Source: CAD feature listing. Evaluate the final solid. Frame: model axes, mm. A direction names the side the tool comes from. Coordinates: 2 decimals unless noted, no trailing zeros. Order: outer loops, then holes, each group sorted by start corner. A loop starts at its lowest first (then second) coordinate and runs counter-clockwise, first axis right, second up. Notation, with made-up numbers: (-30.75, 74) -> (-19.75, 74) arc R31 cw to (-19.75, 112) -> close; hole circle Ø4 at (43, 71.25). An arc over 180 degrees is marked (long way). Write item = value, one per line. Start each with the question number.
Item 1: Section query B-B (x = -25). Output: boundary loops of the cut face in (y, z), then the cut area to 3 significant figures.
Item 2: Contact query for flat-ended pins moving along their axis: pin 1 (6 mm diameter, centred on x = -17, y = 3, fed in from +Z); pin 2 (10 mm diameter, centred on x = -20, z = 10, fed in from +Y); pin 3 (2 mm diameter, centred on x = -26.5, y = 14, fed in from -Z); pin 4 (12 mm diameter, centred on x = -16.5, y = -53.5, fed in from -Z). Output: stop coordinate, or through.
Item 3: Section query C-C (y = -35). Output: boundary loops of the cut face in (x, z).
Item 4: Ray query, line 1 along Y through (x, z) = (-16.75, 6.75); line 2 along X through (y, z) = (-69.3, 10.05); line 3 along Z through (x, y) = (-19.25, 26.5). Return the intervals inside material, ascending. Write a range as [from, to].
Item 5: Section query A-A (z = 6). Output: boundary loops of the cut face in (x, y).
Item 6: Set-up query: faces 1 (the flat face through (-12.21, -34, 10)), 2 (the cylindrical face through (-19.95, -39.68, 1.97)), 3 (the flat face through (-17, -55, 20.1)). Return all of +Z, -Z, +X, -X, +Y, -Y with unobstructed straight access to the full face (end or side cutting, diameter ignored); none if empty.
Item 7: Mould query, pull axis X, two halves, no side actions, for faces 4 (the cylindrical face through (-21.61, -58.31, 22.07)), 5 (the flat face through (-19, -69, 0)), 6 (the flat face through (-29.21, -27, 3)), 7 (the cylindrical face through (-20.41, -45.29, 12.4)). Classes: released by +X, released by -X, zero draft, split by the parting line, or undercut.
Item 8: Section query D-D (y = 0). Output: boundary loops of the cut face in (x, z).
```python
from build123d import *

# Parameters (mm, degrees)
SKETCH_1_W          = 20
SKETCH_1_H          = 90
EXTRUDE_1_DEPTH     = 4
SKETCH_2_W          = 20
SKETCH_2_H          = 4
EXTRUDE_2_DEPTH     = 20.1
SKETCH_3_W          = 20
SKETCH_3_H          = 4
EXTRUDE_3_DEPTH     = 24.1
SKETCH_4_W          = 20
SKETCH_4_H          = 4
EXTRUDE_4_DEPTH     = 20.1
SKETCH_5_R          = 2.6
CUT_EXTRUDE_1_DEPTH = 20
SKETCH_6_R          = 2.6
CUT_EXTRUDE_2_DEPTH = 20
SKETCH_7_R          = 2.6
CUT_EXTRUDE_3_DEPTH = 20
SKETCH_9_R          = 1.6
CUT_EXTRUDE_4_DEPTH = 20
EXTRUDE_5_DEPTH     = 3


with BuildPart() as part:
    # 草图1 → 凸台-拉伸1 (new body)
    with BuildSketch(Plane.XY):
        with Locations((-19.209677061, -2.260885663)):
            Rectangle(SKETCH_1_W, SKETCH_1_H)
    extrude(amount=EXTRUDE_1_DEPTH)

    # 草图2 → 凸台-拉伸2 (add)
    with BuildSketch(Plane.XY.offset(4)):
        with Locations((-19.209677061, -45.260885663)):
            Rectangle(SKETCH_2_W, SKETCH_2_H)
    extrude(amount=EXTRUDE_2_DEPTH)

    # 草图3 → 凸台-拉伸3 (add)
    with BuildSketch(Plane(origin=(0, -47.260885663, 0), x_dir=(-1, 0, 0), z_dir=(0, -1, 0))):
        with Locations((19.209677061, -22.1)):
            Rectangle(SKETCH_3_W, SKETCH_3_H)
    extrude(amount=EXTRUDE_3_DEPTH)

    # 草图4 → 凸台-拉伸4 (add)
    with BuildSketch(Plane(origin=(0, 0, 20.1), x_dir=(-1, 0, 0), z_dir=(0, 0, -1))):
        with Locations((19.209677061, -69.360885663)):
            Rectangle(SKETCH_4_W, SKETCH_4_H)
    extrude(amount=EXTRUDE_4_DEPTH)

    # 草图5 → 切除-拉伸1 (cut)
    with BuildSketch(Plane(origin=(0, -47.260885663, 0), x_dir=(-1, 0, 0), z_dir=(0, -1, 0))):
        with Locations((19.209677061, -10.094759339)):
            Circle(SKETCH_5_R)
    extrude(amount=-CUT_EXTRUDE_1_DEPTH, mode=Mode.SUBTRACT)

    # 草图6 → 切除-拉伸2 (cut)
    with BuildSketch(Plane(origin=(0, 0, 20.1), x_dir=(-1, 0, 0), z_dir=(0, 0, -1))):
        with Locations((19.209677061, -57.310885663)):
            Circle(SKETCH_6_R)
    extrude(amount=-CUT_EXTRUDE_2_DEPTH, mode=Mode.SUBTRACT)

    # 草图7 → 切除-拉伸3 (cut)
    with BuildSketch(Plane(origin=(0, -67.360885663, 0), x_dir=(1, 0, 0), z_dir=(0, 1, 0))):
        with Locations((-19.209677061, -10.05)):
            Circle(SKETCH_7_R)
    extrude(amount=-CUT_EXTRUDE_3_DEPTH, mode=Mode.SUBTRACT)

    # 草图9 → 切除-拉伸4 (cut)
    with BuildSketch(Plane(origin=(0, 0, 0), x_dir=(-1, 0, 0), z_dir=(0, 0, -1))):
        with Locations((19.209677061, 37.739114337)):
            Circle(SKETCH_9_R)
        with Locations((19.209677061, -38.260885663)):
            Circle(SKETCH_9_R)
    extrude(amount=-CUT_EXTRUDE_4_DEPTH, mode=Mode.SUBTRACT)

    # 草图10 → 凸台-拉伸5 (add)
    with BuildSketch(Plane(origin=(-9.209677061, 0, 0), x_dir=(0, 0, -1), z_dir=(1, 0, 0))):
        Polygon((-4, -11.848280973), (-24.1, -43.260885663), (-4, -43.260885663), align=None)
    extrude(amount=-EXTRUDE_5_DEPTH)


solid = part.part
```
Computed:
q1.outline = (-71.36, 0) -> (-67.36, 0) -> (-67.36, 20.1) -> (-47.26, 20.1) -> (-47.26, 0) -> (42.74, 0) -> (42.74, 4) -> (-43.26, 4) -> (-43.26, 24.1) -> (-71.36, 24.1) -> close
q1.area = 617 mm^2
q2.pin_1 = 4
q2.pin_2 = -43.26
q2.pin_3 = 0
q2.pin_4 = 20.1
q3.outline = (-29.21, 0) -> (-9.21, 0) -> (-9.21, 18.81) -> (-12.21, 18.81) -> (-12.21, 4) -> (-29.21, 4) -> close
q4.line_1 = [-71.36, -67.36], [-47.26, -43.26]
q4.line_2 = [-29.21, -21.81], [-16.61, -9.21]
q4.line_3 = [0, 4]
q5.outline = (-29.21, -71.36) -> (-9.21, -71.36) -> (-9.21, -67.36) -> (-29.21, -67.36) -> close; (-29.21, -47.26) -> (-9.21, -47.26) -> (-9.21, -14.97) -> (-12.21, -14.97) -> (-12.21, -43.26) -> (-29.21, -43.26) -> close
q6.face_1 = +Z, -X, +Y
q6.face_2 = +Z, -Z
q6.face_3 = -Z, +X, -X
q7.face_4 = undercut
q7.face_5 = zero draft
q7.face_6 = released by -X
q7.face_7 = undercut
q8.outline = (-29.21, 0) -> (-9.21, 0) -> (-9.21, 4) -> (-29.21, 4) -> close
